Geometry: final body of the model. Coordinates: model frame, mm. A direction names the side the tool comes from. Round coordinates to 2 decimals unless told otherwise and drop trailing zeros. Loops run counter-clockwise (first coordinate to the right, second up) from the corner with the lowest first, then second, coordinate; pieces in that order, holes last. Notation, with made-up numbers: M 87,34.5 L 91,34.5 A24 cw 91,47.5 Z; hole C -7,-0.75 d5. An arc over 180 degrees is marked long. Return JSON: item names as keys, results as strings.
from build123d import *

# Parameters (mm, degrees)
SKETCH1_W                                      = 146.05
SKETCH1_H                                      = 127
BOSS_EXTRUDE2_DEPTH                            = 4.7625
SKETCH2_R                                      = 14.2875
SKETCH2_R_2                                    = 11.1125
CUT_EXTRUDE1_DEPTH                             = 5.7625
CSK_FOR_M6_FLAT_HEAD_MACHINE_SCREW1_AT_2_COUNT = 2
CSK_FOR_M6_FLAT_HEAD_MACHINE_SCREW1_AT_2_PITCH = 89.21849584
CSK_FOR_M6_FLAT_HEAD_MACHINE_SCREW1_AT_3_COUNT = 2
CSK_FOR_M6_FLAT_HEAD_MACHINE_SCREW1_AT_3_PITCH = 67.750719553
CSK_FOR_M6_FLAT_HEAD_MACHINE_SCREW1_AT_4_COUNT = 2
CSK_FOR_M6_FLAT_HEAD_MACHINE_SCREW1_AT_4_PITCH = 67.750719553
F_10_CLEARANCE_HOLE2_D                         = 5.1054
FILLET2_R                                      = 9.525
F_6_32_TAPPED_HOLE1_D                          = 2.7051
SKETCH11_R                                     = 6.35
CUT_EXTRUDE2_DEPTH                             = 5.7625
FILLET28_R                                     = 4.7625


with BuildPart() as part:
    # Sketch1 → Boss-Extrude2 (new body)
    with BuildSketch(Plane(origin=(0, 0, 0), x_dir=(0, 0, -1), z_dir=(1, 0, 0))):
        with Locations((73.025, 63.5)):
            Rectangle(SKETCH1_W, SKETCH1_H)
    extrude(amount=BOSS_EXTRUDE2_DEPTH)

    # Sketch2 → Cut-Extrude1 (cut, through all)
    with BuildSketch(Plane(origin=(4.7625, 0, 0), x_dir=(0, 0, -1), z_dir=(1, 0, 0))):
        with Locations((90.633575625, 51.809624375)):
            Circle(SKETCH2_R)
        with Locations((31.75, 76.2)):
            Circle(SKETCH2_R_2)
        with Locations((66.2432, 76.2)):
            Circle(SKETCH2_R_2)
    extrude(amount=-CUT_EXTRUDE1_DEPTH, mode=Mode.SUBTRACT)

    # Sketch4 → CSK for M6 Flat Head Machine Screw1 (revolve, cut)
    with BuildSketch(Plane(origin=(4.7625, 96.809624375, -90.633575625), x_dir=(0, 0, -1), z_dir=(0, 1, 0))):
        Polygon((0, 0), (0, 4.7625), (3.3, 4.7625), (3.3, 3), (6.3, 0), align=None)
    csk_for_m6_flat_head_machine_screw1 = revolve(axis=Axis((11.1125, 96.809624375, -90.633575625), (-1, 0, 0)), mode=Mode.SUBTRACT)

    # CSK for M6 Flat Head Machine Screw1 at 2: CSK for M6 Flat Head Machine Screw1 ×2
    with Locations(*[Vector(0, -0.991946784, -0.126655352) * (i * CSK_FOR_M6_FLAT_HEAD_MACHINE_SCREW1_AT_2_PITCH) for i in range(1, CSK_FOR_M6_FLAT_HEAD_MACHINE_SCREW1_AT_2_COUNT)]):
        add(csk_for_m6_flat_head_machine_screw1, mode=Mode.SUBTRACT)

    # CSK for M6 Flat Head Machine Screw1 at 3: CSK for M6 Flat Head Machine Screw1 ×2
    with Locations(*[Vector(0, -0.752759533, 0.658295591) * (i * CSK_FOR_M6_FLAT_HEAD_MACHINE_SCREW1_AT_3_PITCH) for i in range(1, CSK_FOR_M6_FLAT_HEAD_MACHINE_SCREW1_AT_3_COUNT)]):
        add(csk_for_m6_flat_head_machine_screw1, mode=Mode.SUBTRACT)

    # CSK for M6 Flat Head Machine Screw1 at 4: CSK for M6 Flat Head Machine Screw1 ×2
    with Locations(*[Vector(0, -0.752759533, -0.658295591) * (i * CSK_FOR_M6_FLAT_HEAD_MACHINE_SCREW1_AT_4_PITCH) for i in range(1, CSK_FOR_M6_FLAT_HEAD_MACHINE_SCREW1_AT_4_COUNT)]):
        add(csk_for_m6_flat_head_machine_screw1, mode=Mode.SUBTRACT)

    # #10 Clearance Hole2 (through all)
    with Locations(Plane(origin=(4.7625, 0, 0), x_dir=(0, 0, -1), z_dir=(1, 0, 0))):
        with Locations((111.125, 35.934624375), (9.525, 103.879624375), (111.125, 80.384624375), (9.525, 51.809624375)):
            Hole(F_10_CLEARANCE_HOLE2_D / 2)

    # Fillet2
    fillet2_edges = [part.edges().sort_by_distance(p)[0] for p in [
        (2.38125, 127, 0),
        (2.38125, 127, -146.05),
        (2.38125, 0, -146.05),
        (2.38125, 0, 0),
    ]]
    fillet(fillet2_edges, radius=FILLET2_R)

    # #6-32 Tapped Hole1 (through all)
    with Locations(Plane.ZY):
        with Locations((-31.75, 76.2), (-19.05, 57.15), (-44.45, 57.15), (-44.45, 95.25), (-19.05, 95.25)):
            Hole(F_6_32_TAPPED_HOLE1_D / 2)

    # Sketch11 → Cut-Extrude2 (cut, through all)
    with BuildSketch(Plane(origin=(4.7625, 0, 0), x_dir=(0, 0, -1), z_dir=(1, 0, 0))):
        with Locations((9.525, 77.844624375)):
            Circle(SKETCH11_R)
        with Locations((63.5, 51.809624375)):
            Circle(SKETCH11_R)
        with BuildLine():
            Line((19.05, 103.879624375), (42.6466, 103.879624375))
            ThreePointArc((42.6466, 103.879624375), (45.223903728, 98.77185942), (50.863690659, 97.81031861))
            Line((50.863690659, 97.81031861), (86.914095809, 108.900446097))
            ThreePointArc((86.914095809, 108.900446097), (93.741933528, 109.07178614), (99.663642833, 105.66854001))
            Line((99.663642833, 105.66854001), (117.92431938, 87.055072709))
            ThreePointArc((117.92431938, 87.055072709), (120.050883489, 77.059834316), (111.903571622, 70.89149785))
            ThreePointArc((111.903571622, 70.89149785), (116.471992165, 64.012364056), (118.882504918, 56.114112587))
            Line((118.882504918, 56.114112587), (133.328001666, 58.315274614))
            ThreePointArc((133.328001666, 58.315274614), (140.589870378, 57.26966829), (146.05, 52.369156655))
            Line((146.05, 52.369156655), (146.05, 127))
            Line((146.05, 127), (0, 127))
            Line((0, 127), (0, 103.879624375))
            ThreePointArc((0, 103.879624375), (9.525, 113.404624375), (19.05, 103.879624375))
        make_face()
        with BuildLine():
            Line((112.343545309, 26.487890954), (114.479631034, 9.927954891))
            ThreePointArc((114.479631034, 9.927954891), (114.040060834, 4.641448277), (111.471533621, 0))
            Line((111.471533621, 0), (146.05, 0))
            Line((146.05, 0), (146.05, 39.250092095))
            ThreePointArc((146.05, 39.250092095), (140.778077608, 34.439444176), (133.741328545, 33.247948585))
            Line((133.741328545, 33.247948585), (120.583495012, 34.811015408))
            ThreePointArc((120.583495012, 34.811015408), (117.893928842, 29.233338877), (112.343545309, 26.487890954))
        make_face()
        with BuildLine():
            Line((91.611269982, 0.997134634), (67.316588768, 35.291490433))
            Line((67.316588768, 35.291490433), (53.0614742, 35.291490433))
            ThreePointArc((53.0614742, 35.291490433), (39.259729687, 35.126108511), (33.522617739, 47.680034163))
            ThreePointArc((33.522617739, 47.680034163), (26.054731603, 48.198311785), (18.97770782, 50.638326004))
            ThreePointArc((18.97770782, 50.638326004), (8.938236412, 42.302714599), (0, 51.809624375))
            Line((0, 51.809624375), (0, 0))
            Line((0, 0), (92.395617628, 0))
            ThreePointArc((92.395617628, 0), (91.990935768, 0.488728475), (91.611269982, 0.997134634))
        make_face()
    extrude(amount=-CUT_EXTRUDE2_DEPTH, mode=Mode.SUBTRACT)

    # Fillet28
    fillet28_edges = [part.edges().sort_by_distance(p)[0] for p in [
        (2.38125, 103.879624375, -19.05),
        (2.38125, 103.879624375, -42.6466),
        (2.38125, 70.89149785, -111.903571622),
        (2.38125, 56.114112587, -118.882504918),
        (2.38125, 39.250092095, -146.05),
        (2.38125, 52.369156655, -146.05),
        (2.38125, 34.811015408, -120.583495012),
        (2.38125, 26.487890954, -112.343545309),
        (2.38125, 0, -111.471533621),
        (2.38125, 0, -92.395617628),
        (2.38125, 35.291490433, -67.316588768),
        (2.38125, 35.291490433, -53.0614742),
        (2.38125, 47.680034163, -33.522617739),
        (2.38125, 50.638326004, -18.97770782),
    ]]
    fillet(fillet28_edges, radius=FILLET28_R)


solid = part.part
Q1. Material intervals for L1, parallel to Y at x = 0.5, z = -135; L2, parallel to Y at x = 1, z = -20; L3, parallel to Y at x = 1.2, z = -63.5, sorted ascending.
Determined:
{"L1": "y = 33.16 to 42.52, 49.1 to 58.46", "L2": "y = 48.83 to 56.19, 58.11 to 94.29, 96.21 to 104.94", "L3": "y = 35.29 to 45.46, 58.16 to 65.43, 86.97 to 101.7"}
Q2. Pull-direction query (Z, two-part tool) for faces 1 (the flat face through (2, 77, 0)), 2 (the cylindrical face through (2.41, 79.64, -120.62)), 3 (the cylindrical face through (2.415, 34.368, -40.638)); classes: pulls with the +Z half, pulls with the -Z half, needs draft (parallel to the pull), parting line crosses it, or undercut.
Determined:
{"face 1": "pulls with the +Z half", "face 2": "pulls with the -Z half", "face 3": "undercut"}
Q3. Section query A-A (y = 76.2). Output: boundary loops of the cut face in (x, z).
Determined:
{"outline": "M 0,-119.68 L 4.76,-119.68 L 4.76,-77.36 L 0,-77.36 Z; M 0,-55.13 L 4.76,-55.13 L 4.76,-42.86 L 0,-42.86 Z; M 0,-20.64 L 4.76,-20.64 L 4.76,-15.66 L 0,-15.66 Z; M 0,-3.39 L 4.76,-3.39 L 4.76,0 L 0,0 Z"}
Q4. Pin query (flat end, axial travel): pin 1 (1.5 mm diameter, centred on x = 0.5, z = -22.5, fed in from +Y); pin 2 (8.5 mm diameter, centred on y = 45.81, z = -135.23, fed in from +X); pin 3 (1.5 mm diameter, centred on x = 3, z = -32.5, fed in from -Y). Return the tip coordinate at first contact, or that it passes through.
Determined:
{"pin 1": "stops at y = 104.05", "pin 2": "stops at x = 2.72", "pin 3": "stops at y = 44.81"}
Q5. Reachability of faces 4 (the cylindrical face through (2.35, 104.78, -20.21)), 5 (the flat face through (2, 35.291, -60)), 6 (the cylindrical face through (2.348, 25.45, -113.383)) from +Z, -Z, +X, -X, +Y, -Y: full face, straight path, thin tool, end or side. Return the list, or none.
Determined:
{"face 4": "+X, -X, +Y", "face 5": "+X, -X, -Y", "face 6": "-Z, +X, -X"}
Q6. Section query B-B (x = 3.85). State how many separate pieces and enclosed holes the cut face has, plus the area to 3 significant figures.
Determined:
{"separate pieces": "1", "enclosed holes": "17", "area": "7,480 mm^2"}
